Input: part model. Units: mm. Frame: model coordinates. A direction names the side the tool comes from. Round coordinates to 2 decimals unless told otherwise and drop trailing zeros. Write each loop counter-clockwise with the first axis right and the second up, starting at its lowest first coordinate (ties: lowest second). Pieces come first, ordered by that corner, then holes. Notation, with made-up numbers: M 13.5,71.25 L 32.5,71.25 A24 cw 32.5,83.25 Z; hole C 51,49 d1. An arc over 180 degrees is marked long. Use one line per item in the form item = value. Start each with the question number.
```python
from build123d import *

# Parameters (mm, degrees)
BOSS_EXTRUDE1_DEPTH = 1.5
CUT_EXTRUDE5_START  = -3.25
CUT_EXTRUDE5_DEPTH  = 3.25
CUT_EXTRUDE6_START  = -54
CUT_EXTRUDE6_DEPTH  = 3.15


# Read off the part's stored shape, not the designer's step: Cut-Extrude6
with BuildPart() as part:
    # Sketch1 → Boss-Extrude1 (new body)
    with BuildSketch(Plane.XY):
        Polygon((47.6, -15), (47.6, 0), (50.75, 0), (50.75, 1.4), (42.5, 1.4), (5.1, 1.4), (-3.25, 1.4), (-3.25, 0), (0, 0), (0, -15), (-3.2, -15), (-3.2, -43.3), (50.8, -43.3), (50.8, -15), align=None)
    extrude(amount=BOSS_EXTRUDE1_DEPTH)

    # Sketch3 → Cut-Extrude5 (cut)
    with BuildSketch(Plane.ZY.offset(3.25).offset(CUT_EXTRUDE5_START)):
        with BuildLine():
            Line((0.75, 1.4), (0, 1.4))
            Line((0, 1.4), (0, 0))
            Line((0, 0), (0.75, 0))
            ThreePointArc((0.75, 0), (0.05, 0.7), (0.75, 1.4))
        make_face()
        with BuildLine():
            Line((1.5, 1.4), (0.75, 1.4))
            ThreePointArc((0.75, 1.4), (1.45, 0.7), (0.75, 0))
            Line((0.75, 0), (1.5, 0))
            Line((1.5, 0), (1.5, 1.4))
        make_face()
    extrude(amount=CUT_EXTRUDE5_DEPTH, mode=Mode.SUBTRACT)

    # Cut-Extrude6 outline → Cut-Extrude6 (cut)
    with BuildSketch(Plane.ZY.offset(3.25).offset(CUT_EXTRUDE6_START)):
        with BuildLine():
            ThreePointArc((0.75, 1.4), (1.45, 0.7), (0.75, 0))
            Line((0.75, 0), (1.5, 0))
            Line((1.5, 0), (1.5, 1.4))
            Line((1.5, 1.4), (0.75, 1.4))
        make_face()
        with BuildLine():
            ThreePointArc((0.75, 0), (0.05, 0.7), (0.75, 1.4))
            Line((0.75, 1.4), (0, 1.4))
            Line((0, 1.4), (0, 0))
            Line((0, 0), (0.75, 0))
        make_face()
    extrude(amount=CUT_EXTRUDE6_DEPTH, mode=Mode.SUBTRACT)


solid = part.part
```
Item 1: Draft query along Y for faces 1 (the face through (24, 1.4, 1)), 2 (the face through (47.6, -7, 1)), 3 (the face through (-3.2, -29, 1)). Return one class per face: +Y half, -Y half, draft (parallel to the pull), parting line (faces both ways), or undercut.
Item 2: Ray query, line 1 (X direction, y = -37, z = 1.05); line 2 (Y direction, x = -1, z = 0.2); line 3 (X direction, y = -6, z = 1.2). Return the intervals inside material, ascending. Write a range as from..to.
Item 3: First-contact query: pin 1 (0.7 mm diameter, centred on y = 0.5, z = 1, fed in from +X). Flat tip, straight axial feed; report the tip coordinate or a pass-through.
Item 4: Cut plane B-B (y = -4). Output: boundary loops of the cut face in (x, z), plus the area to 3 significant figures.
Item 5: Reachability of faces 4 (the face through (49.197, 0.852, 1.433)), 5 (the face through (50.75, 1, 1)), 6 (the face through (-2, -15, 1)), 7 (the face through (49, -15, 1)) from +Z, -Z, +X, -X, +Y, -Y: full face, straight path, thin tool, end or side. Return the list, or none.
Item 6: Cut plane A-A (z = 0.4). Output: boundary loops of the cut face in (x, y), plus the area to 3 significant figures.
Final values:
q1.face_1 = +Y half
q1.face_2 = undercut
q1.face_3 = draft
q2.line_1 = -3.2..50.8
q2.line_2 = -43.3..-15, 0.27..1.13
q2.line_3 = 0..47.6
q3.pin_1 = 50.75
q4.outline = M 0,0 L 47.6,0 L 47.6,1.5 L 0,1.5 Z
q4.area = 71.4 mm^2
q5.face_4 = +X
q5.face_5 = +Z, -Z, +X, +Y
q5.face_6 = +Z, -Z, -X
q5.face_7 = +Z, -Z, +X
q6.outline = M -3.25,0.09 L 0,0.09 L 0,-15 L -3.2,-15 L -3.2,-43.3 L 50.8,-43.3 L 50.8,-15 L 47.6,-15 L 47.6,0.09 L 50.75,0.09 L 50.75,1.31 L 47.6,1.31 L 47.6,1.4 L 0,1.4 L 0,1.31 L -3.25,1.31 Z
q6.area = 2,320 mm^2
